Part print with two shaded views. Sizes in mm from the minimum x, y, z corner. Coordinates: 2 decimals unless noted, no trailing zeros. Loops run counter-clockwise (first coordinate to the right, second up) from the corner with the lowest first, then second, coordinate; pieces in that order, holes last. Notation, with made-up numbers: (32, -27) -> (80, -27) arc R16 ccw to (80, 3) -> close; hole circle Ø8 at (59.5, 70). An arc over 180 degrees is marked (long way). Write each question's results on one line, items separated by ' | '.
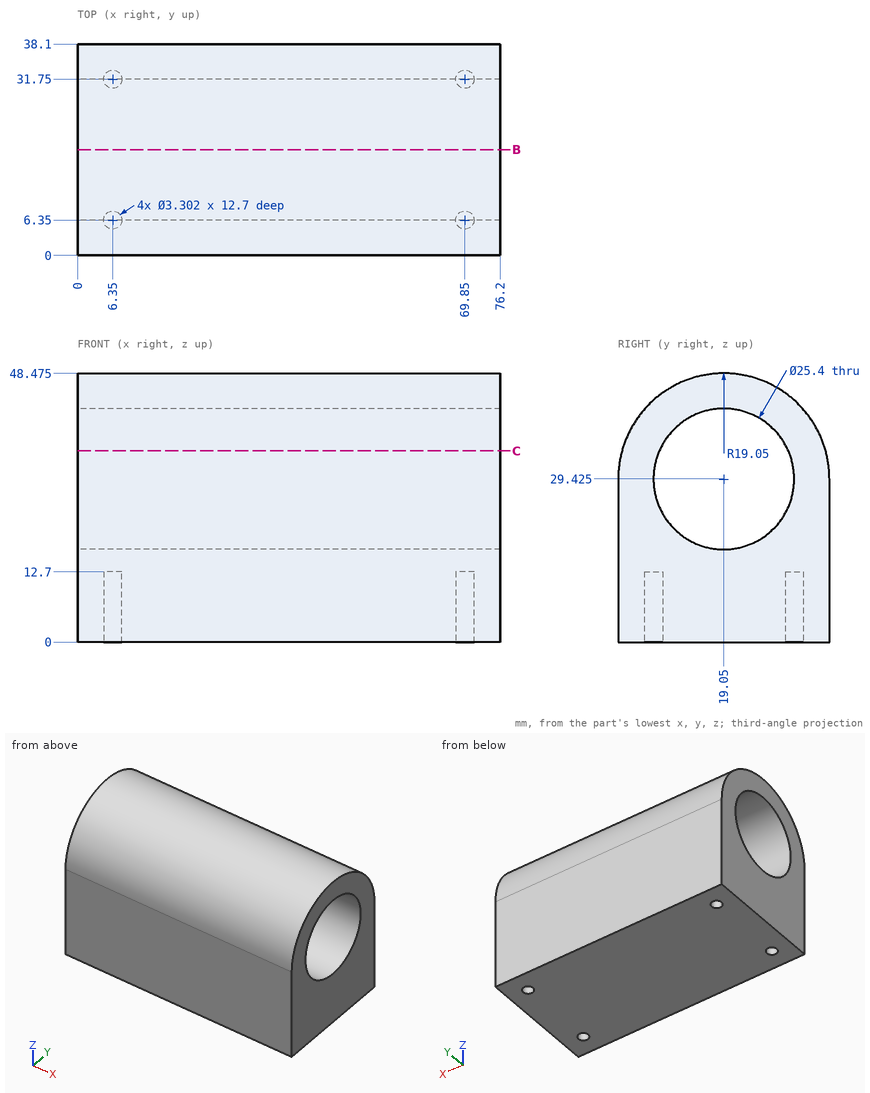
Q1. Cut at C-C on z = 34.5. Write the cut outline in (x, y), and give its area (3 significant figures).
Results are:
outline: (0, 0.69) -> (76.2, 0.69) -> (76.2, 7.41) -> (0, 7.41) -> close; (0, 30.69) -> (76.2, 30.69) -> (76.2, 37.41) -> (0, 37.41) -> close | area: 1,020 mm^2
Q2. Wall check: L1, parallel to Y at x = 6.35, z = 9.25; L2, parallel to X at y = 31.75, z = 7; L3, parallel to Y at x = 69, z = 2 (1 decimal). Give the ranges that are in metal, low to high. Write a range as from..to.
Results are:
L1: 0..4.7, 8..30.1, 33.4..38.1 | L2: 0..4.7, 8..68.2, 71.5..76.2 | L3: 0..4.9, 7.8..30.3, 33.2..38.1
Q3. Drop flat-ended pins along their axis: pin 1 (1 mm diameter, centred on x = 69.5, y = 31.5, fed in from -Z); pin 2 (1 mm diameter, centred on x = 11.5, z = 34.5, fed in from -Y); pin 3 (4 mm diameter, centred on x = 69.85, y = 6.35, fed in from +Z) (1 decimal). Give the stop position or say it passes through.
Results are:
pin 1: z = 12.7 | pin 2: y = 0.56 | pin 3: z = 45.2
Q4. Cut at B-B on y = 19.05. Write the cut outline in (x, z) (1 decimal).
Results are:
outline: (0, 0) -> (76.2, 0) -> (76.2, 16.7) -> (0, 16.7) -> close; (0, 42.1) -> (76.2, 42.1) -> (76.2, 48.5) -> (0, 48.5) -> close
